from build123d import *

# Parameters (mm, degrees)
F1_DEPTH = 1
F2_R     = 6.322095
F3_DEPTH = 25


with BuildPart() as f1:
    # F0 (on Top) → F1 (new body)
    with BuildSketch(Plane.XY):
        Polygon((50, 75), (-18.058607, 75), (-50, 13.215269), (-50, -75), (28.098688, -75), (28.098688, -43.112274), (50, 28.602385), (36.704283, 37.858568), (50, 48.314037), (37.486609, 57.025582), align=None)
    extrude(amount=F1_DEPTH)

    # F2 (on face) → F3 (cut)
    with BuildSketch(Plane.XY.offset(1)):
        with Locations((8.059037, 48.924173)):
            Circle(F2_R)
        with BuildLine():
            Line((-20.704884, 10.188761), (-20.704444, 9.23894))
            ThreePointArc((-20.704444, 9.23894), (-20.682059, 9.713861), (-20.704884, 10.188761))
        make_face()
        with BuildLine():
            Line((-20.682059, -39.073944), (-20.704444, 9.23894))
            Line((-20.704444, 9.23894), (-20.704884, 10.188761))
            ThreePointArc((-20.704884, 10.188761), (-25.920939, 14.705834), (-30.682058, 9.711544))
            Line((-30.682058, 9.711544), (-30.682058, -39.076261))
            ThreePointArc((-30.682058, -39.076261), (-25.6809, -44.076261), (-20.682059, -39.073944))
        make_face()
    extrude(amount=-F3_DEPTH, mode=Mode.SUBTRACT)


solid = f1.part
Input: part model. Units: mm. Frame: model coordinates. A direction names the side the tool comes from. Give positions to 0.01 mm unless a question says otherwise; leave off trailing zeros. Loops run counter-clockwise (first coordinate to the right, second up) from the corner with the lowest first, then second, coordinate; pieces in that order, holes last. Notation, with made-up numbers: (-16.5, -18) - (21.5, -18) arc R22 cw to (21.5, 7) - close; hole circle Ø11 at (-19.5, 56.5). An arc over 180 degrees is marked (long way). Use CSV: the item, a comma, the result in double quotes. Start each with the question number.
Item 1: Line query: line 1 (X direction, y = -52.5, z = 0.55); line 2 (Y direction, x = 11, z = 0.3); line 3 (X direction, y = -7.5, z = 0.35). Output: solid intervals per line, ascending.
Item 2: Section D-D on x = 44. Return loops of the section in (y, z), then the cut area to 3 significant figures.
Item 3: Mould query, pull axis Y, two halves, no side actions, for faces 4 (the cylindrical face through (-25.81, 14.71, 0.51)), 5 (the flat face through (43.66, 65.89, 0.49)), 6 (the flat face through (-1, 1, 0)), 7 (the flat face through (38.896, -7.757, 0.493)). Classes: pulls with the +Y half, pulls with the -Y half, needs draft (parallel to the pull), parting line crosses it, or undercut.
Item 4: Section C-C on z = 0.65. Return loops of the section in (x, y).
Item 5: Contact query for flat-ended pins moving along their axis: P1, Ø8, axis at x = 4, y = 39.5, coming from the -Z side; P2, Ø0.5, axis at y = -10.5, z = 0.5, coming from the +X side; P3, Ø11.5, axis at x = 8.06, y = 48.92, coming from the -Z side. Output: stop coordinate, or through.
Item 6: Section A-A on y = 7. Return loops of the section in (x, z), then the cut area to 3 significant figures.
Item 7: Section B-B on x = -26.5. Return loops of the section in (y, z), then the cut area to 3 significant figures.
Item 8: Reachability of faces 1 (the cylindrical face through (-25.791, -44.075, 0.507)), 2 (the flat face through (-1, 1, 1)), 3 (the flat face through (43.445, 33.166, 0.493)) from +Z, -Z, +X, -X, +Y, -Y: full face, straight path, thin tool, end or side. Return the list, or none.
Ans:
1,line 1,"x = -50 to 28.1"
1,line 2,"y = -75 to 43.33, 54.52 to 75"
1,line 3,"x = -50 to -30.68, -20.7 to 38.97"
2,outline,"(8.96, 0) - (32.78, 0) - (32.78, 1) - (8.96, 1) - close; (43.6, 0) - (52.49, 0) - (52.49, 1) - (43.6, 1) - close; (66.38, 0) - (75, 0) - (75, 1) - (66.38, 1) - close"
2,area,"41.3 mm2"
3,face 4,"undercut"
3,face 5,"undercut"
3,face 6,"needs draft"
3,face 7,"pulls with the -Y half"
4,outline,"(-50, -75) - (28.1, -75) - (28.1, -43.11) - (50, 28.6) - (36.7, 37.86) - (50, 48.31) - (37.49, 57.03) - (50, 75) - (-18.06, 75) - (-50, 13.22) - close; hole (-30.68, -39.08) arc R5 ccw to (-20.68, -39.07) - (-20.7, 9.24) arc R5 ccw to (-20.7, 10.19) arc R5 ccw to (-30.68, 9.71) - close; hole circle Ø12.64 at (8.06, 48.92)"
5,P1,"stops at z = 0"
5,P2,"stops at x = 38.13"
5,P3,"passes through"
6,outline,"(-50, 0) - (-30.68, 0) - (-30.68, 1) - (-50, 1) - close; (-20.7, 0) - (43.4, 0) - (43.4, 1) - (-20.7, 1) - close"
6,area,"83.4 mm2"
7,outline,"(-75, 0) - (-44.01, 0) - (-44.01, 1) - (-75, 1) - close; (14.64, 0) - (58.67, 0) - (58.67, 1) - (14.64, 1) - close"
7,area,"75.0 mm2"
8,face 1,"+Z, -Z"
8,face 2,"+Z, +X, -X, +Y, -Y"
8,face 3,"+Z, -Z, +X"
